```python
from build123d import *

# Parameters (mm, degrees)
CHAMFER_1_SIZE      = 1
CUT_EXTRUDE_1_DEPTH = 2.5
CHAMFER_2_SIZE      = 1


with BuildPart() as part:
    # 草图1 → 旋转1 (revolve)
    with BuildSketch(Plane.XY):
        Polygon((-58.75, 0), (-58.75, 9), (-39.25, 9), (-38.85, 8.6), (-36.85, 8.6), (-36.85, 10.6), (-37.25, 11), (-37.25, 19.5), (-21.25, 19.5), (-21.25, 11), (-21.65, 10.6), (-21.65, 8.6), (-19.65, 8.6), (-19.25, 9), (24.75, 9), (24.75, 8), (58.75, 8), (58.75, 0), align=None)
    revolve(axis=Axis((58.75, 0, 0), (-1, 0, 0)))

    # 倒角1
    chamfer_1_edges = [part.edges().sort_by_distance(p)[0] for p in [
        (-58.75, -9, 0),
    ]]
    chamfer(chamfer_1_edges, length=CHAMFER_1_SIZE)

    # 草图3 → 切除-拉伸1 (cut, symmetric)
    with BuildSketch(Plane.XY):
        with BuildLine():
            Line((58.75, 5), (33.75, 5))
            ThreePointArc((33.75, 5), (29.877016654, 5.780455543), (26.608571571, 8))
            Line((26.608571571, 8), (26.608571571, 13))
            Line((26.608571571, 13), (58.75, 13))
            Line((58.75, 13), (58.75, 5))
        make_face()
    extrude(amount=CUT_EXTRUDE_1_DEPTH, both=True, mode=Mode.SUBTRACT)

    # 倒角2
    chamfer_2_edges = [part.edges().sort_by_distance(p)[0] for p in [
        (58.75, -8, 0),
    ]]
    chamfer(chamfer_2_edges, length=CHAMFER_2_SIZE)


solid = part.part
```
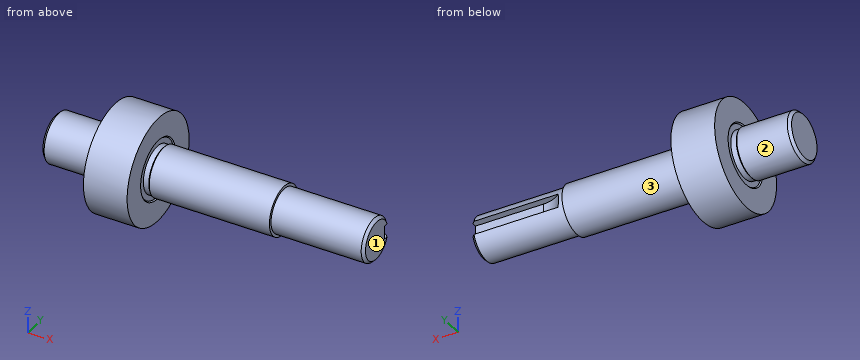
CAD build for the part. Positions are in the model's coordinates, mm. Face numbers are marked on the shaded views. A direction names the side the tool comes from. Give positions to 0.01 mm unless a question says otherwise; leave off trailing zeros. Loops run counter-clockwise (first coordinate to the right, second up) from the corner with the lowest first, then second, coordinate; pieces in that order, holes last. Notation, with made-up numbers: (83, 0) -> (120, 0) arc R21 cw to (120, 26) -> close; hole circle Ø2 at (48.25, 26.25). An arc over 180 degrees is marked (long way). Use a Markdown table: item, result.
1. Which spindle directions (+Z, -Z, +X, -X, +Y, -Y) get a long thin tool onto all of the face, cutting with end or side? Do the marked faces 1, 2 and 3. Say none if no direction does.
Check result:
| item | result |
|---|---|
| face 1 | +Z, -Z, +X, +Y, -Y |
| face 2 | -X |
| face 3 | +X |
2. Slice it at B-B (z = 14). List the corners of the cut face in (x, y).
Check result:
| item | result |
|---|---|
| outline | (-37.25, -13.57) -> (-21.25, -13.57) -> (-21.25, 13.57) -> (-37.25, 13.57) -> close |
3. Slice it at A-A (x = 49). List the corners of the cut face in (y, z), plus the area to 3 significant figures.
Check result:
| item | result |
|---|---|
| outline | (5, -2.5) -> (5, 2.5) -> (7.6, 2.5) arc R8 ccw (long way) to (7.6, -2.5) -> close |
| area | 187 mm^2 |
4. Slice it at C-C (x = -9). List the corners of the cut face in (y, z).
Check result:
| item | result |
|---|---|
| outline | circle Ø18 at (0, 0) |
5. Wall check: L1, parallel to Y at x = -24, z = 17.5; L2, parallel to X at y = -2.5, z = -11; L3, parallel to X at y = -10.5, z = -1. Give the ranges that are in metal, low to high. Write a range as [from, to].
Check result:
| item | result |
|---|---|
| L1 | y = [-8.6, 8.6] |
| L2 | x = [-37.25, -21.25] |
| L3 | x = [-36.85, -21.65] |
6. Flat gauge pins, fed straight in: pin 1 (3 mm diameter, centred on x = 38, z = -4.5, fed in from +Y); pin 2 (4 mm diameter, centred on y = 14.5, z = 4, fed in from +X); pin 3 (1 mm diameter, centred on x = 14, z = 10, fed in from -Y); pin 4 (6 mm diameter, centred on x = -9.5, z = 2, fed in from -Y). Where does each tip first touch, or does it go through?
Check result:
| item | result |
|---|---|
| pin 1 | stops at y = 7.42 |
| pin 2 | stops at x = -21.25 |
| pin 3 | passes through |
| pin 4 | stops at y = -9 |
